```python
from build123d import *

# Parameters (mm, degrees)
F0_W     = 10
F0_H     = 1.5875
F0_W_2   = 1.5875
F0_H_2   = 10
F1_DEPTH = 1.5875


# Not quite as in the source:
# - a length typed as a fraction of an inch, garbled in the dataset ("3 / 203.2 mm" for 3/8 in), is restored


with BuildPart() as f1:
    # F0 (on Right) → F1 (new body)
    with BuildSketch(Plane.YZ):
        Polygon((15.5766666667, 44.4233333333), (-44.4233333333, -15.5766666667), (-34.4233333333, -15.5766666667), (-24.4233333333, -15.5766666667), (-4.4233333333, -15.5766666667), (5.5766666667, -15.5766666667), (15.5766666667, -15.5766666667), (15.5766666667, -5.5766666667), (15.5766666667, 4.4233333333), (15.5766666667, 24.4233333333), (15.5766666667, 34.4233333333), align=None)
        with Locations((-29.4233333333, -16.3704166667)):
            Rectangle(F0_W, F0_H)
        with Locations((16.3704166667, 29.4233333333)):
            Rectangle(F0_W_2, F0_H_2)
        with Locations((0.5766666667, -16.3704166667)):
            Rectangle(F0_W, F0_H)
        with Locations((16.3704166667, -0.5766666667)):
            Rectangle(F0_W_2, F0_H_2)
    extrude(amount=F1_DEPTH)


solid = f1.part
```
The listing builds one solid part. Answer for the finished solid, in the listing's coordinates (mm). A direction names the side the tool comes from. Round coordinates to 2 decimals unless told otherwise and drop trailing zeros. Write each loop counter-clockwise with the first axis right and the second up, starting at its lowest first coordinate (ties: lowest second). Pieces come first, ordered by that corner, then holes. Notation, with made-up numbers: (49, 73) -> (71, 73) arc R15 cw to (71, 97) -> close; hole circle Ø9 at (34, 61.5). An arc over 180 degrees is marked (long way). Use CSV: the item, a comma, the result in double quotes. Start each with the question number.
(1) Which of the six approach directions +Z, -Z, +X, -X, +Y, -Y give full straight-line access (tool end or side, diameter ignored) to faces 1 (the face through (1, -39, -15.577)), 2 (the face through (1, 11, -15.577)), 3 (the face through (1, -24.423, -16)), 4 (the face through (1, 15.577, 14))?
(2) Each of these flat-tipped pins is pushed along its axis until it touches: pin 1 (0.5 mm diameter, centred on x = 1, y = -13, fed in from -Z); pin 2 (0.8 mm diameter, centred on x = 0.5, y = 16.5, fed in from -Z); pin 3 (0.8 mm diameter, centred on x = 0.5, z = 15.5, fed in from +Y). Where does it stop, or does it pass through?
(3) Section A-A on x = 0.4 is taken. Give the vertices of the cut face in (y, z).
(4) Section B-B on y = -26.5 is taken. Give the vertices of the cut face in (x, z), then the cut area to 3 significant figures.
(5) The mould has two halves that part along X. Classify faces 5 (the face through (1, -29, -17.164)), 6 (the face through (1.588, -7, 7)), 7 (the face through (0, -7, 7)): released by +X, released by -X, zero draft, split by the parting line, or undercut.
(6) Section C-C on z = 28 is taken. Give the vertices of the cut face in (x, y), then the cut area to 3 significant figures.
(7) Consider L1, parallel to Z at x = 1.5, y = -37.5; L2, parallel to Z at x = 1.25, y = 11; L3, parallel to Y at x = 1.2, z = 40.5. Determine where each line is inside the solid, lowest interval first. Write a range as from..to.
A:
1,face 1,"-Z, +X, -X, -Y"
1,face 2,"-Z, +X, -X, +Y"
1,face 3,"-Z, +X, -X"
1,face 4,"+X, -X, +Y"
2,pin 1,"stops at z = -15.58"
2,pin 2,"stops at z = -5.58"
2,pin 3,"stops at y = 15.58"
3,outline,"(-44.42, -15.58) -> (-34.42, -15.58) -> (-34.42, -17.16) -> (-24.42, -17.16) -> (-24.42, -15.58) -> (-4.42, -15.58) -> (-4.42, -17.16) -> (5.58, -17.16) -> (5.58, -15.58) -> (15.58, -15.58) -> (15.58, -5.58) -> (17.16, -5.58) -> (17.16, 4.42) -> (15.58, 4.42) -> (15.58, 24.42) -> (17.16, 24.42) -> (17.16, 34.42) -> (15.58, 34.42) -> (15.58, 44.42) -> close"
4,outline,"(0, -17.16) -> (1.59, -17.16) -> (1.59, 2.35) -> (0, 2.35) -> close"
4,area,"31.0 mm²"
5,face 5,"zero draft"
5,face 6,"released by +X"
5,face 7,"released by -X"
6,outline,"(0, -0.85) -> (1.59, -0.85) -> (1.59, 17.16) -> (0, 17.16) -> close"
6,area,"28.6 mm²"
7,L1,"z = -15.58..-8.65"
7,L2,"z = -15.58..39.85"
7,L3,"y = 11.65..15.58"
